Part model, mm, in its own coordinate system. Face numbers are marked on the shaded views. A direction names the side the tool comes from. Give positions to 0.01 mm unless a question says otherwise; leave off trailing zeros. Loops run counter-clockwise (first coordinate to the right, second up) from the corner with the lowest first, then second, coordinate; pieces in that order, holes last. Notation, with made-up numbers: (15, 12) -> (20, 12) arc R28 cw to (20, 35) -> close; hole circle Ø8 at (29.5, 86). An arc over 180 degrees is marked (long way). One line per question, with ' | ' between items.
```python
from build123d import *

# Parameters (mm, degrees)
F1_DEPTH    = 25.4
F2_T        = -2.54
F3_T2_ANGLE = 202.0417037701
F3_T4_ANGLE = 119.7204573229
F3_T6_ANGLE = 119.7204573229
F5_DEPTH    = 2.54


# Not quite as in the source:
# - a fillet or chamfer that OpenCascade refuses, or shapes differently, is made with other operations: its cross-section is extruded or revolved along the edge and cut away or added


with BuildPart() as f1:
    # F0 (on Top) → F1 (new body)
    with BuildSketch(Plane.XY):
        with BuildLine():
            ThreePointArc((-53.34, 0), (-15.6229242915, -15.6229242915), (0, -53.34))
            ThreePointArc((0, -53.34), (15.6229242915, -15.6229242915), (53.34, 0))
            ThreePointArc((53.34, 0), (0, 53.34), (-53.34, 0))
        make_face()
    extrude(amount=F1_DEPTH)

    # F2
    f2_openings = [f1.faces().sort_by_distance(p)[0] for p in [
        (0, 15.223138, 25.4),
    ]]
    offset(amount=F2_T, openings=f2_openings)

    # F3: chamfer of 2.286 x 3.9594681461 on 3 edges, made by hand

    # F3_s1 → F3_t2 (revolve, cut)
    with BuildSketch(Plane(origin=(0, 0, 0), x_dir=(0, 0, 1), z_dir=(-0.1911662303, -0.9815576766, 0))):
        Polygon((21.4405318539, -53.34), (25.4, -51.054), (25.4, -53.34), align=None)
    revolve(axis=Axis((0, 0, 25.4), (0, 0, 1)), revolution_arc=F3_T2_ANGLE, mode=Mode.SUBTRACT)

    # F3_s3 → F3_t4 (revolve, cut)
    with BuildSketch(Plane(origin=(-61.3926477335, -11.9419473665, 0), x_dir=(0, 0, 1), z_dir=(-0.9816019423, -0.190938804, 0))):
        Polygon((21.4405318539, 11.1660282003), (25.4, 13.4520282003), (25.4, 11.1660282003), align=None)
    revolve(axis=Axis((-53.34, -53.34, 25.4), (0, 0, -1)), revolution_arc=F3_T4_ANGLE, mode=Mode.SUBTRACT)

    # F3_s5 → F3_t6 (revolve, cut)
    with BuildSketch(Plane(origin=(21.6984854346, -64.0579906243, 0), x_dir=(0, 0, 1), z_dir=(0.3208259227, -0.9471381775, 0))):
        Polygon((21.4405318539, 19.9325043289), (25.4, 22.2185043289), (25.4, 19.9325043289), align=None)
    revolve(axis=Axis((53.34, -53.34, 25.4), (0, 0, -1)), revolution_arc=F3_T6_ANGLE, mode=Mode.SUBTRACT)

    # F4 (on face) → F5 (cut, through all)
    with BuildSketch(Plane(origin=(0, 0, 0), x_dir=(1, 0, 0), z_dir=(0, 0, -1))):
        with BuildLine():
            ThreePointArc((-46.6093067615, -5.9693067615), (0, -46.99), (46.6093067615, -5.9693067615))
            ThreePointArc((46.6093067615, -5.9693067615), (19.1861227863, 4.3868716907), (0, 26.5493206506))
            ThreePointArc((0, 26.5493206506), (-19.1861227863, 4.3868716907), (-46.6093067615, -5.9693067615))
        make_face()
    extrude(amount=-F5_DEPTH, mode=Mode.SUBTRACT)


solid = f1.part
```
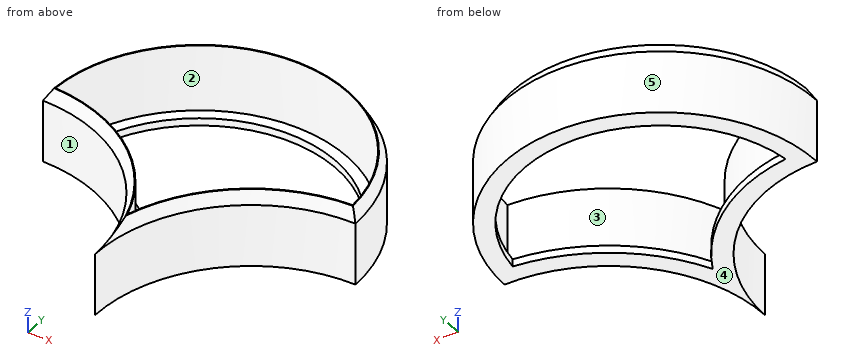
1) Drill centre lines: line 1 (Y direction, x = -4, z = 10.75); line 2 (X direction, y = -29.5, z = 18.5); line 3 (Y direction, x = -16.5, z = 7). Where is each one in solid material? Low to high.
Found:
line 1: -33.07 to -27.11, 50.64 to 53.19 | line 2: -5.62 to -2.8, 2.8 to 5.62 | line 3: -14.77 to -11.32, 48.05 to 50.72
2) Tool access for the marked faces 1 and 2: list every direction of +Z, -Z, +X, -X, +Y, -Y with a clear straight run to the whole face (end or side of a thin tool).
Found:
face 1: +Z, -Z, -X, -Y | face 2: +Z
3) Saw through at A-A (z = 7.5). Give the cut face in (x, y).
Found:
outline: (-53.34, 0) arc R53.34 cw to (0, -53.34) arc R53.34 cw to (53.34, 0) arc R53.34 ccw to start; hole (-50.74, 2.48) arc R55.88 cw to (0, -36.68) arc R55.88 cw to (50.74, 2.48) arc R50.8 ccw to start
4) Pin check, flat tips, straight feed: P1, Ø3, axis at y = -40, z = 4, coming from the -X side; P2, Ø1.5, axis at x = -18, z = 9.5, coming from the -Y side; P3, Ø8, axis at x = -19, z = 10.5, coming from the +Y side. Stop position of each tip, or through.
Found:
P1: x = -2.11 | P2: y = -14.06 | P3: y = 51.19
5) Pull direction Y, two halves, no side cores. Call the marked faces 3, 4 and 5: pulls with the +Y half, pulls with the -Y half, needs draft (parallel to the pull), parting line crosses it, or undercut.
Found:
face 3: undercut | face 4: needs draft | face 5: pulls with the +Y half
